from build123d import *

# Parameters (mm, degrees)
SKETCH2_W                               = 292.1
SKETCH2_H                               = 292.1
BOSS_EXTRUDE1_DEPTH                     = 12.7
F_6_5_6_5_DIAMETER_HOLE1_D              = 6.5
CBORE_FOR_M5_HEX_HEAD_BOLT1_D           = 5.5
CBORE_FOR_M5_HEX_HEAD_BOLT1_CBORE_D     = 12.24
CBORE_FOR_M5_HEX_HEAD_BOLT1_CBORE_DEPTH = 3.58
CBORE_FOR_M4_SBHCS1_D                   = 4.5
CBORE_FOR_M4_SBHCS1_CBORE_D             = 8.6
CBORE_FOR_M4_SBHCS1_CBORE_DEPTH         = 2.2


with BuildPart() as part:
    # Sketch2 → Boss-Extrude1 (new body)
    with BuildSketch(Plane(origin=(0, 0, 0), x_dir=(1, 0, 0), z_dir=(0, 1, 0))):
        Rectangle(SKETCH2_W, SKETCH2_H)
    extrude(amount=BOSS_EXTRUDE1_DEPTH)

    # Ø6.5 (6.5) Diameter Hole1 (through all)
    with Locations(Plane(origin=(0, 12.7, 0), x_dir=(1, 0, 0), z_dir=(0, 1, 0))):
        with Locations((-125, 125), (125, 125), (125, -125), (-125, -125)):
            Hole(F_6_5_6_5_DIAMETER_HOLE1_D / 2)

    # CBORE for M5 Hex Head Bolt1 (through all)
    with Locations(Plane(origin=(0, 12.7, 0), x_dir=(1, 0, 0), z_dir=(0, 1, 0))):
        with Locations((-73.5, -15), (-111.5, 15), (-111.5, -15), (-73.5, 15)):
            cbore_for_m5_hex_head_bolt1 = CounterBoreHole(CBORE_FOR_M5_HEX_HEAD_BOLT1_D / 2, CBORE_FOR_M5_HEX_HEAD_BOLT1_CBORE_D / 2, CBORE_FOR_M5_HEX_HEAD_BOLT1_CBORE_DEPTH)

    # Mirror1: CBORE for M5 Hex Head Bolt1 across plane
    add(cbore_for_m5_hex_head_bolt1.mirror(Plane(origin=(0, 0, 0), x_dir=(0, 0, 1), z_dir=(1, 0, 0))), mode=Mode.SUBTRACT)

    # CBORE for M4 SBHCS1 (through all)
    with Locations(Plane(origin=(0, 12.7, 0), x_dir=(1, 0, 0), z_dir=(0, 1, 0))):
        with Locations((56.500001429, 10), (56.500001429, -10.0000005)):
            CounterBoreHole(CBORE_FOR_M4_SBHCS1_D / 2, CBORE_FOR_M4_SBHCS1_CBORE_D / 2, CBORE_FOR_M4_SBHCS1_CBORE_DEPTH)


solid = part.part
For this review, take the finished solid that the model builds, in its own axes (mm). A direction names the side the tool comes from. Round coordinates to 2 decimals unless told otherwise and drop trailing zeros. Answer as CSV lines item,"result".
(1) Mouldability with a two-part tool opening along X and no side actions: class faces 1 (the face through (-72, 9.12, -12)), 2 (the face through (-2, 12.7, -2)) as +X half, -X half, draft (parallel to the pull), parting line (faces both ways), or undercut.
Checked values:
face 1,"undercut"
face 2,"draft"
(2) Wall thickness on line 1 (Z direction, x = 73.5, y = 3.5); line 2 (Z direction, x = 111.5, y = 10.55); line 3 (X direction, y = 1, z = 127): over which ranges is each line inside the solid? List them lowest first.
Checked values:
line 1,"z = -146.05 to -17.75, -12.25 to 12.25, 17.75 to 146.05"
line 2,"z = -146.05 to -21.12, -8.88 to 8.88, 21.12 to 146.05"
line 3,"x = -146.05 to -127.56, -122.44 to 122.44, 127.56 to 146.05"
(3) Tool access review of faces 3 (the face through (-108.9, 9.12, 16.3)), 4 (the face through (-126.5, 6.261, 127.883)): name each direction out of +Z, -Z, +X, -X, +Y, -Y from which nothing blocks a thin tool from reaching the whole face with its end or side.
Checked values:
face 3,"+Y"
face 4,"+Y, -Y"
(4) Insertion check: P1, Ø7, axis at x = -111.5, z = 15, coming from the -Y side; P2, Ø7, axis at x = 56.5, z = 10, coming from the +Y side; P3, Ø6, axis at x = -113.5, z = -13, coming from the +Y side; P4, Ø4.5, axis at x = 111.5, z = 15, coming from the +Y side. Each pin has a flat end and moves straight along its axis. Give the tip position at first contact, or say it passes through.
Checked values:
P1,"stops at y = 0"
P2,"stops at y = 10.5"
P3,"stops at y = 9.12"
P4,"passes through"
